from build123d import *

# Parameters (mm, degrees)
SKETCH2_R                = 7.62
BOSS_EXTRUDE1_DEPTH      = 34.29
BOSS_EXTRUDE2_DEPTH      = 17.145
BOSS_EXTRUDE2_DEPTH_BACK = 17.145
SKETCH3_R                = 7.62
FILLET1_R                = 1.27


with BuildPart() as part:
    # Sketch2 → Boss-Extrude1 (new body)
    with BuildSketch(Plane.XY):
        Circle(SKETCH2_R)
    extrude(amount=BOSS_EXTRUDE1_DEPTH)

    # Sketch3 → Boss-Extrude2 (add, two sides: drawn at the far end of the back side and taken through both)
    with BuildSketch(Plane(origin=(0, 0, 0), x_dir=(0, 0, -1), z_dir=(1, 0, 0)).offset(-BOSS_EXTRUDE2_DEPTH_BACK)):
        with Locations((-17.145, 0)):
            Circle(SKETCH3_R)
    extrude(amount=BOSS_EXTRUDE2_DEPTH + BOSS_EXTRUDE2_DEPTH_BACK)

    # Fillet1
    fillet1_edges = [part.edges().sort_by_distance(p)[0] for p in [
        (-7.62, 0, 0),
        (-7.62, 0, 34.29),
        (-17.145, 0, 24.765),
        (17.145, 0, 24.765),
    ]]
    fillet(fillet1_edges, radius=FILLET1_R)


solid = part.part
Geometry: final body of the model. Coordinates: model frame, mm. A direction names the side the tool comes from. Give positions to 0.01 mm unless a question says otherwise; leave off trailing zeros. Loops run counter-clockwise (first coordinate to the right, second up) from the corner with the lowest first, then second, coordinate; pieces in that order, holes last. Notation, with made-up numbers: M 60.5,60 L 117.5,60 A31 cw 117.5,91 Z; hole C -1.75,9.25 d11. An arc over 180 degrees is marked long. Put each result on its own line as item: value. Start each with the question number.
1) Cut plane A-A (y = 0). Output: boundary loops of the cut face in (x, z) (3 decimals), then the cut area to 3 significant figures.
2) Cut plane B-B (z = 31). Output: boundary loops of the cut face in (x, y).
3) Ray query, line 1 along X through (y, z) = (-0.25, 26); line 2 along X through (y, z) = (-2.75, 23). Return the intervals inside material, ascending.
4) Cut plane C-C (x = -9.5). Output: boundary loops of the cut face in (y, z) (3 decimals), then the cut area to 3 significant figures.
5) Contact query for flat-ended pins moving along their axis: pin 1 (6 mm diameter, centred on x = 4, z = 26.5, fed in from -Y); pin 2 (1 mm diameter, centred on x = 4.5, z = 8, fed in from +Y); pin 3 (10 mm diameter, centred on x = 9, z = 22.5, fed in from +Y). Output: stop coordinate, or through.
6) Access query for faces 1 (the cylindrical face through (-9.81, 5.15, 22.76)), 2 (the cylindrical face through (9.59, 0.335, 24.758)), 3 (the cylindrical face through (-5.616, 5.15, 7.332)). Directions: +Z, -Z, +X, -X, +Y, -Y. A direction counts if a zero-diameter tool reaches every point of the face in a straight line with its end or side. Return the directions, or none.
Verdict:
1. outline: M -17.145,10.795 A1.27 ccw -15.875,9.525 L -7.62,9.525 L -7.62,1.27 A1.27 ccw -6.35,0 L 6.35,0 A1.27 ccw 7.62,1.27 L 7.62,9.525 L 15.875,9.525 A1.27 ccw 17.145,10.795 L 17.145,23.495 A1.27 ccw 15.875,24.765 L 7.62,24.765 L 7.62,33.02 A1.27 ccw 6.35,34.29 L -6.35,34.29 A1.27 ccw -7.62,33.02 L -7.62,24.765 L -15.875,24.765 A1.27 ccw -17.145,23.495 Z
1. area: 810 mm2
2. outline: C 0,0 d15.24
3. line 1: -7.62 to 7.62
3. line 2: -17.14 to 17.14
4. outline: C 0,17.145 d15.24
4. area: 182 mm2
5. pin 1: y = -7.55
5. pin 2: y = 6.49
5. pin 3: y = 7.61
6. face 1: -X
6. face 2: +X
6. face 3: -Z
